The listing builds one solid part. Answer for the finished solid, in the listing's coordinates (mm). Round coordinates to 2 decimals unless told otherwise and drop trailing zeros. Write each loop counter-clockwise with the first axis right and the second up, starting at its lowest first coordinate (ties: lowest second). Pieces come first, ordered by that corner, then holes. Notation, with made-up numbers: M 40,51 L 60,51 A7 ccw 60,64 Z; hole C 8.25,78.25 d4. An arc over 180 degrees is marked long. Write each question's results on one line, items separated by ' | '.
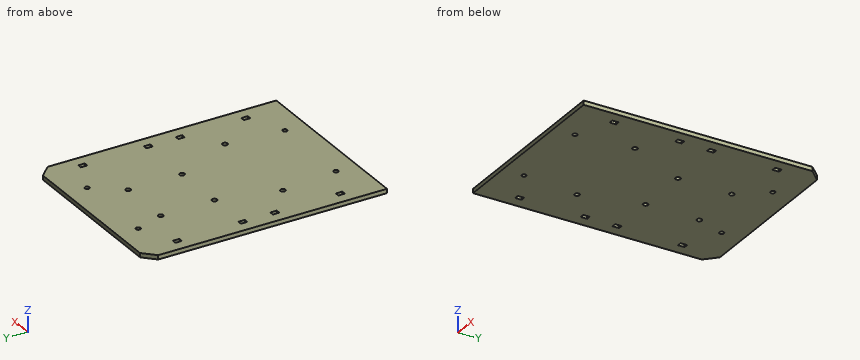
from build123d import *

# Parameters (mm, degrees)
SKETCH_1_R      = 1.6
SKETCH_1_R_2    = 1.75
SKETCH_1_W      = 3
SKETCH_1_H      = 4.6
EXTRUDE_1_DEPTH = 3


with BuildPart() as part:
    # ｽｹｯﾁ1 → ﾎﾞｽ - 押し出し1 (new body)
    with BuildSketch(Plane.XY):
        Polygon((0, 162), (8, 170), (122, 170), (130, 162), (130, 0), (0, 0), align=None)
        with Locations((35, 155)):
            Circle(SKETCH_1_R, mode=Mode.SUBTRACT)
        with Locations((95, 155)):
            Circle(SKETCH_1_R, mode=Mode.SUBTRACT)
        with Locations((35, 15)):
            Circle(SKETCH_1_R, mode=Mode.SUBTRACT)
        with Locations((95, 15)):
            Circle(SKETCH_1_R, mode=Mode.SUBTRACT)
        with Locations((41.9, 135)):
            Circle(SKETCH_1_R_2, mode=Mode.SUBTRACT)
        with Locations((80, 135)):
            Circle(SKETCH_1_R_2, mode=Mode.SUBTRACT)
        with Locations((41.9, 96.9)):
            Circle(SKETCH_1_R_2, mode=Mode.SUBTRACT)
        with Locations((80, 96.9)):
            Circle(SKETCH_1_R_2, mode=Mode.SUBTRACT)
        with Locations((31, 55)):
            Circle(SKETCH_1_R_2, mode=Mode.SUBTRACT)
        with Locations((99, 55)):
            Circle(SKETCH_1_R_2, mode=Mode.SUBTRACT)
        with Locations((9.5, 142.7)):
            Rectangle(SKETCH_1_W, SKETCH_1_H, mode=Mode.SUBTRACT)
        with Locations((120.5, 142.7)):
            Rectangle(SKETCH_1_W, SKETCH_1_H, mode=Mode.SUBTRACT)
        with Locations((9.5, 27.3)):
            Rectangle(SKETCH_1_W, SKETCH_1_H, mode=Mode.SUBTRACT)
        with Locations((120.5, 27.3)):
            Rectangle(SKETCH_1_W, SKETCH_1_H, mode=Mode.SUBTRACT)
        with Locations((9.5, 96.3)):
            Rectangle(SKETCH_1_W, SKETCH_1_H, mode=Mode.SUBTRACT)
        with Locations((120.5, 96.3)):
            Rectangle(SKETCH_1_W, SKETCH_1_H, mode=Mode.SUBTRACT)
        with Locations((9.5, 73.7)):
            Rectangle(SKETCH_1_W, SKETCH_1_H, mode=Mode.SUBTRACT)
        with Locations((120.5, 73.7)):
            Rectangle(SKETCH_1_W, SKETCH_1_H, mode=Mode.SUBTRACT)
    extrude(amount=EXTRUDE_1_DEPTH)


solid = part.part
1) Section C-C (x = 80) is taken. Determine the outline of the cut face in (y, z).
Return value:
outline: M 0,0 L 95.15,0 L 95.15,3 L 0,3 Z; M 98.65,0 L 133.25,0 L 133.25,3 L 98.65,3 Z; M 136.75,0 L 170,0 L 170,3 L 136.75,3 Z
2) Section A-A (y = 55) is taken. Determine the outline of the cut face in (x, z), then the cut area to 3 significant figures.
Return value:
outline: M 0,0 L 29.25,0 L 29.25,3 L 0,3 Z; M 32.75,0 L 97.25,0 L 97.25,3 L 32.75,3 Z; M 100.75,0 L 130,0 L 130,3 L 100.75,3 Z | area: 369 mm²
3) Find the intervals of material crossed by line 1 (X direction, y = 135, z = 1.8); line 2 (Y direction, x = 80, z = 2); line 3 (Y direction, x = 35, z = 0.8), in increasing order.
Return value:
line 1: 0 to 40.15, 43.65 to 78.25, 81.75 to 130 | line 2: 0 to 95.15, 98.65 to 133.25, 136.75 to 170 | line 3: 0 to 13.4, 16.6 to 153.4, 156.6 to 170
4) Section B-B (x = 99) is taken. Determine the outline of the cut face in (y, z).
Return value:
outline: M 0,0 L 53.25,0 L 53.25,3 L 0,3 Z; M 56.75,0 L 170,0 L 170,3 L 56.75,3 Z
5) Each of these flat-tipped pins is pushed along its axis until it touches: pin 1 (5 mm diameter, centred on x = 69, y = 59.5, fed in from -Z); pin 2 (2.5 mm diameter, centred on x = 95, y = 15, fed in from -Z). Where does it stop, or does it pass through?
Return value:
pin 1: z = 0 | pin 2: through
